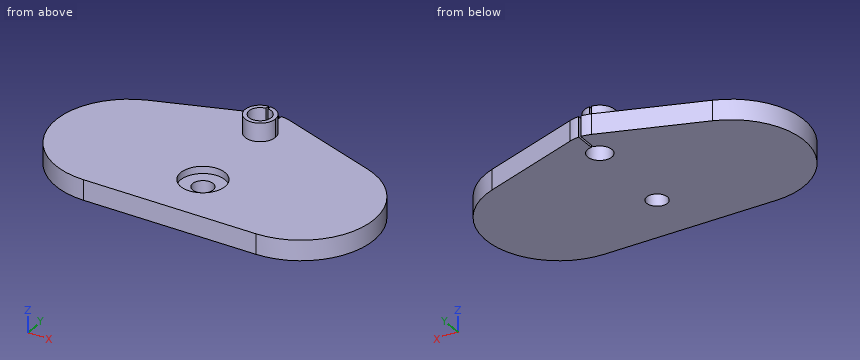
```python
from build123d import *

# Parameters (mm, degrees)
SKETCH1_R           = 6
SKETCH1_R_2         = 11
BOSS_EXTRUDE1_DEPTH = 10
SKETCH2_R           = 7.5
SKETCH2_R_2         = 5.5
BOSS_EXTRUDE2_DEPTH = 9
SKETCH3_R           = 11
SKETCH3_R_2         = 5.1
BOSS_EXTRUDE3_DEPTH = 6.5
SKETCH4_W           = 1
SKETCH4_H           = 19
CUT_EXTRUDE1_DEPTH  = 14


with BuildPart() as part:
    # Sketch1 → Boss-Extrude1 (new body)
    with BuildSketch(Plane.XY):
        with BuildLine():
            Line((54.380555702, -18.011258697), (5.266349667, -0.891540079))
            ThreePointArc((5.266349667, -0.891540079), (0, 0), (-5.266349667, -0.891540079))
            Line((-5.266349667, -0.891540079), (-54.380555702, -18.011258697))
            ThreePointArc((-54.380555702, -18.011258697), (-78.08863349, -58.119798033), (-42.5, -88.19))
            Line((-42.5, -88.19), (42.5, -88.19))
            ThreePointArc((42.5, -88.19), (78.08863349, -58.119798033), (54.380555702, -18.011258697))
        make_face()
        with Locations((0, -16)):
            Circle(SKETCH1_R, mode=Mode.SUBTRACT)
        with Locations((0, -61.697507746)):
            Circle(SKETCH1_R_2, mode=Mode.SUBTRACT)
    extrude(amount=BOSS_EXTRUDE1_DEPTH)

    # Sketch2 → Boss-Extrude2 (add)
    with BuildSketch(Plane.XY.offset(10)):
        with Locations((0, -16)):
            Circle(SKETCH2_R)
        with Locations((0, -16)):
            Circle(SKETCH2_R_2, mode=Mode.SUBTRACT)
    extrude(amount=BOSS_EXTRUDE2_DEPTH)

    # Sketch3 → Boss-Extrude3 (add)
    with BuildSketch(Plane(origin=(0, 0, 0), x_dir=(-1, 0, 0), z_dir=(0, 0, -1))):
        with Locations((0, -61.697507746)):
            Circle(SKETCH3_R)
        with Locations((0, -61.697507746)):
            Circle(SKETCH3_R_2, mode=Mode.SUBTRACT)
    extrude(amount=-BOSS_EXTRUDE3_DEPTH)

    # Sketch4 → Cut-Extrude1 (cut)
    with BuildSketch(Plane(origin=(0, 1.81, 0), x_dir=(-1, 0, 0), z_dir=(0, -1, 0))):
        with Locations((0, -9.5)):
            Rectangle(SKETCH4_W, SKETCH4_H)
    extrude(amount=CUT_EXTRUDE1_DEPTH, mode=Mode.SUBTRACT)


solid = part.part
```
Geometry check sheet. Reference: the model listing, model coordinates, mm. Round coordinates to 2 decimals unless told otherwise and drop trailing zeros. Order: outer loops, then holes, each group sorted by start corner. A loop starts at its lowest first (then second) coordinate and runs counter-clockwise, first axis right, second up. Notation, with made-up numbers: (76, 51) -> (82, 51) arc R7 cw to (82, 60) -> close; hole circle Ø5 at (43, -26). An arc over 180 degrees is marked (long way). Return JSON: item names as keys, results as strings. Group by question number.
Q1. Material ranges on probe 1 along X at (y, z) = (-16, 16.75); probe 2 along Z at (x, y) = (7, -4.5); probe 3 along Y at (x, z) = (0, 14.75), recorded low to high. Write a range as from..to.
Q2. Section check A-A, the plane y = -65. Record the boundary of the cut face in (x, z), plus the area to 3 significant figures.
Q3. Gauge pin test, flat ends, axial feed: pin 1 (8 mm diameter, centred on y = -73.5, z = 5.5, fed in from +X); pin 2 (12.5 mm diameter, centred on x = 0, y = -16, fed in from +Z); pin 3 (3 mm diameter, centred on x = 52.5, z = 2, fed in from -Y); pin 4 (3 mm diameter, centred on x = -25.5, z = 7, fed in from +Y). Record the tip position at first contact, or that the pin passes through.
Q4. Section check B-B, the plane z = 13.25. Record the boundary of the cut face in (x, y).
Q5. Section check C-C, the plane x = -28. Record the boundary of the cut face in (y, z), plus the area to 3 significant figures.
Numbers:
{
 "1": {"probe 1": "-7.5..-5.5, 5.5..7.5", "probe 2": "0..10", "probe 3": "-23.5..-21.5"},
 "2": {"outline": "(-76.21, 0) -> (-3.89, 0) -> (-3.89, 6.5) -> (-10.49, 6.5) -> (-10.49, 10) -> (-76.21, 10) -> close; (3.89, 0) -> (76.21, 0) -> (76.21, 10) -> (10.49, 10) -> (10.49, 6.5) -> (3.89, 6.5) -> close", "area": "1,400 mm^2"},
 "3": {"pin 1": "x = 74.12", "pin 2": "z = 19", "pin 3": "y = -87.17", "pin 4": "y = -7.42"},
 "4": {"outline": "(-0.5, -10.52) -> (-0.5, -8.52) arc R7.5 ccw (long way) to (0.5, -8.52) -> (0.5, -10.52) arc R5.5 cw (long way) to start"},
 "5": {"outline": "(-88.19, 0) -> (-8.82, 0) -> (-8.82, 10) -> (-88.19, 10) -> close", "area": "794 mm^2"}
}
